Build history of the part. All positions in model axes, mm. Round coordinates to 2 decimals unless told otherwise and drop trailing zeros. Use a Markdown table: item, result.
Autodesk Inventor part; units mm, degrees
ref_plane "YZ Plane" through (0, 0, 0) normal (1, 0, 0) x (0, 1, 0)
ref_plane "XZ Plane" through (0, 0, 0) normal (0, 1, 0) x (-1, 0, 0)
ref_plane "XY Plane" through (0, 0, 0) normal (0, 0, 1) x (1, 0, 0)
sketch "Sketch1" plane through (0, 0, 0) normal (0, 0, 1) x (1, 0, 0)
  line L0 (0, 0) -> (286, 0)
  arc A0 (271.0494, 3.9199) -> (0, 50) centre (-140.2784, -1595.3524) ccw
  arc A1 (273.6055, 6.3591) -> (0, 53.0109) centre (-140.2784, -1595.3524) ccw
  arc A2 (286, 0) -> (273.6055, 6.3591) centre (265.6617, -24.3829) ccw
  arc A3 (280.1558, 0) -> (271.0494, 3.9199) centre (263.3021, -26.6152) ccw
  line L1 (-3, 0) -> (0, 0)
  line L2 (0, 50) -> (0, 53.0109)
  dimension "d0" = 286
  dimension "d1" = 50
  dimension "d2" = 3
revolve "Revolution1" add sketch "Sketch1" angle 360 about axis through (0, 0, 0) along (1, 0, 0)
sketch "Sketch2" plane through (0, 0, 0) normal (-1, 0, 0) x (0, 0, 1)
  circle A0 centre (0, 0) radius 50
  line L0 (0, 50) -> (2, 50)
  line L1 (2, 50) -> (2, 41)
  line L2 (2, 41) -> (0, 41)
  line L3 (0, 50) -> (-2, 50)
  line L4 (-2, 50) -> (-2, 41)
  line L5 (-2, 41) -> (0, 41)
  line L6 (-43.3013, 25) -> (-42.3013, 26.7321)
  line L7 (-42.3013, 26.7321) -> (-34.507, 22.2321)
  line L8 (-34.507, 22.2321) -> (-35.507, 20.5)
  line L9 (-43.3013, 25) -> (-44.3013, 23.2679)
  line L10 (-44.3013, 23.2679) -> (-36.507, 18.7679)
  line L11 (-36.507, 18.7679) -> (-35.507, 20.5)
  line L12 (-43.3013, -25) -> (-44.3013, -23.2679)
  line L13 (-44.3013, -23.2679) -> (-36.507, -18.7679)
  line L14 (-36.507, -18.7679) -> (-35.507, -20.5)
  line L15 (-43.3013, -25) -> (-42.3013, -26.7321)
  line L16 (-42.3013, -26.7321) -> (-34.507, -22.2321)
  line L17 (-34.507, -22.2321) -> (-35.507, -20.5)
  line L18 (0, -50) -> (-2, -50)
  line L19 (-2, -50) -> (-2, -41)
  line L20 (-2, -41) -> (0, -41)
  line L21 (0, -50) -> (2, -50)
  line L22 (2, -50) -> (2, -41)
  line L23 (2, -41) -> (0, -41)
  line L24 (43.3013, -25) -> (42.3013, -26.7321)
  line L25 (42.3013, -26.7321) -> (34.507, -22.2321)
  line L26 (34.507, -22.2321) -> (35.507, -20.5)
  line L27 (43.3013, -25) -> (44.3013, -23.2679)
  line L28 (44.3013, -23.2679) -> (36.507, -18.7679)
  line L29 (36.507, -18.7679) -> (35.507, -20.5)
  line L30 (43.3013, 25) -> (44.3013, 23.2679)
  line L31 (44.3013, 23.2679) -> (36.507, 18.7679)
  line L32 (36.507, 18.7679) -> (35.507, 20.5)
  line L33 (43.3013, 25) -> (42.3013, 26.7321)
  line L34 (42.3013, 26.7321) -> (34.507, 22.2321)
  line L35 (34.507, 22.2321) -> (35.507, 20.5)
  point P0 (-44.2666, -23.2479)
  point P1 (-42.2666, -26.712)
  point P2 (0, -41)
  point P3 (-2, -49.96)
  point P4 (2, -49.96)
  point P5 (42.2666, -26.712)
  point P6 (44.2666, -23.2479)
  point P7 (-42.2666, 26.712)
  point P8 (-44.2666, 23.2479)
  point P9 (44.2666, 23.2479)
  point P10 (42.2666, 26.712)
  point P11 (2, 49.96)
  point P12 (-2, 49.96)
  dimension "d4" = 2
  dimension "d5" = 9
  dimension "d6" = 2
  dimension "d9" = 360
extrude "Extrusion1" add sketch "Sketch2" against normal up to next contours L31 L32 L35 L34 A0 | A0 L25 L26 L29 L28 | L1 L2 L5 L4 A0 | A0 L19 L20 L23 L22 | L7 L8 L11 L10 A0 | A0 L13 L14 L17 L16
sketch "Sketch4" plane through (0, 0, 0) normal (-1, 0, 0) x (0, 0, 1)
  circle A0 centre (0, 0) radius 3.9199
  circle A1 centre (0, 0) radius 50
  line L0 (0, 50) -> (1.25, 50)
  line L1 (1.25, 50) -> (1.25, 46)
  line L2 (1.25, 46) -> (0, 46)
  line L3 (0, 50) -> (-1.25, 50)
  line L4 (-1.25, 50) -> (-1.25, 46)
  line L5 (-1.25, 46) -> (0, 46)
  line L6 (-43.3013, 25) -> (-42.6763, 26.0825)
  line L7 (-42.6763, 26.0825) -> (-39.2122, 24.0825)
  line L8 (-39.2122, 24.0825) -> (-39.8372, 23)
  line L9 (-43.3013, 25) -> (-43.9263, 23.9175)
  line L10 (-43.9263, 23.9175) -> (-40.4622, 21.9175)
  line L11 (-40.4622, 21.9175) -> (-39.8372, 23)
  line L12 (-43.3013, -25) -> (-43.9263, -23.9175)
  line L13 (-43.9263, -23.9175) -> (-40.4622, -21.9175)
  line L14 (-40.4622, -21.9175) -> (-39.8372, -23)
  line L15 (-43.3013, -25) -> (-42.6763, -26.0825)
  line L16 (-42.6763, -26.0825) -> (-39.2122, -24.0825)
  line L17 (-39.2122, -24.0825) -> (-39.8372, -23)
  line L18 (0, -50) -> (-1.25, -50)
  line L19 (-1.25, -50) -> (-1.25, -46)
  line L20 (-1.25, -46) -> (0, -46)
  line L21 (0, -50) -> (1.25, -50)
  line L22 (1.25, -50) -> (1.25, -46)
  line L23 (1.25, -46) -> (0, -46)
  line L24 (43.3013, -25) -> (42.6763, -26.0825)
  line L25 (42.6763, -26.0825) -> (39.2122, -24.0825)
  line L26 (39.2122, -24.0825) -> (39.8372, -23)
  line L27 (43.3013, -25) -> (43.9263, -23.9175)
  line L28 (43.9263, -23.9175) -> (40.4622, -21.9175)
  line L29 (40.4622, -21.9175) -> (39.8372, -23)
  line L30 (43.3013, 25) -> (43.9263, 23.9175)
  line L31 (43.9263, 23.9175) -> (40.4622, 21.9175)
  line L32 (40.4622, 21.9175) -> (39.8372, 23)
  line L33 (43.3013, 25) -> (42.6763, 26.0825)
  line L34 (42.6763, 26.0825) -> (39.2122, 24.0825)
  line L35 (39.2122, 24.0825) -> (39.8372, 23)
  point P0 (-42.6627, 26.0747)
  point P1 (-43.9127, 23.9097)
  point P2 (-43.9127, -23.9097)
  point P3 (-42.6627, -26.0747)
  point P4 (0, -46)
  point P5 (-1.25, -49.9844)
  point P6 (1.25, -49.9844)
  point P7 (42.6627, -26.0747)
  point P8 (43.9127, -23.9097)
  point P9 (43.9127, 23.9097)
  point P10 (42.6627, 26.0747)
  point P11 (1.25, 49.9844)
  point P12 (-1.25, 49.9844)
  dimension "d29" = 1.25
  dimension "d30" = 4
  dimension "d31" = 1.25
  dimension "d34" = 360
extrude "Extrusion3" add sketch "Sketch4" along normal blind 17 contours L31 L32 L35 L34 A1 | A1 L25 L26 L29 L28 | L1 L2 L5 L4 A1 | A1 L19 L20 L23 L22 | L7 L8 L11 L10 A1 | A1 L13 L14 L17 L16
equation "\"BendRadius\" = Thickness"
equation "\"BendReliefWidth\" = Thickness"
equation "\"BendReliefDepth\" = 0.5 * Thickness"
equation "\"CornerReliefSize\" = 4 * Thickness"
equation "\"MinimumRemnant\" = 2 * Thickness"
equation "\"TransitionRadius\" = BendRadius"
equation "\"JacobiRadiusSize\" = BendRadius"
equation "\"GapSize\" = Thickness"
properties part number "Nosecone(finale)tip"
Q1. Drop flat-ended pins along their axis: pin 1 (5 mm diameter, centred on x = 171, z = -12, fed in from -Y); pin 2 (1.5 mm diameter, centred on x = 114, y = -11, fed in from +Z); pin 3 (1.5 mm diameter, centred on x = 168.5, z = 11.5, fed in from +Y). Give the stop position or say it passes through.
Results found:
| item | result |
|---|---|
| pin 1 | stops at y = -27.98 |
| pin 2 | stops at z = 37.98 |
| pin 3 | stops at y = 27.94 |
Q2. Probe line 1 (Z direction, x = 27.5, y = -4); line 2 (Y direction, x = 159, z = 8.5); line 3 (Y direction, x = 29, z = -18). List the from-to ranges inside material, lowest first.
Results found:
| item | result |
|---|---|
| line 1 | z = -50.28 to -47.25, 47.25 to 50.28 |
| line 2 | y = -30.51 to -27.33, 27.33 to 30.51 |
| line 3 | y = -46.95 to -43.71, 43.71 to 46.95 |
Q3. Pull direction Y, two halves, no side cores. Call faces 1 (the face through (31.01, -20.54, -39.58)), 2 (the face through (31.01, 20.54, -39.58)): pulls with the +Y half, pulls with the -Y half, needs draft (parallel to the pull), parting line crosses it, or undercut.
Results found:
| item | result |
|---|---|
| face 1 | undercut |
| face 2 | undercut |
